```python
from build123d import *

# Parameters (mm, degrees)
SKETCH_1_R                   = 3.85
EXTRUDE_1_DEPTH              = 8
EXTRUDE_1_2_DEPTH            = 8
EXTRUDE_1_3_DEPTH            = 8
SKETCH_1_3_R                 = 28.3
SKETCH_1_3_R_2               = 0.5
EXTRUDE_2_DEPTH              = 3
SKETCH_2_R                   = 3.2
CUT_EXTRUDE_1_DEPTH          = 41.333360882
HOLE_WIZARD_M2_1_D           = 2.4
HOLE_WIZARD_M2_1_DEPTH       = 3
HOLE_WIZARD_M2_1_CBORE_D     = 5
HOLE_WIZARD_M2_1_CBORE_DEPTH = 1.6
HOLE_WIZARD_M2_1_TIP         = 0.721032743


with BuildPart() as part:
    # Sketch 1 → Extrude 1 (new body)
    with BuildSketch(Plane(origin=(0, 0, 0), x_dir=(1, 0, 0), z_dir=(0, 1, 0))):
        with Locations(Location((0, 14.33, 0), (0, 0, 270))):
            Circle(SKETCH_1_R)
    extrude(amount=EXTRUDE_1_DEPTH)



with BuildPart() as body_2:
    # Sketch 1 → Extrude 1 2 (new body)
    with BuildSketch(Plane(origin=(0, 0, 0), x_dir=(1, 0, 0), z_dir=(0, 1, 0))):
        with Locations(Location((12.410144036, -7.165, 0), (0, 0, 270))):
            Circle(SKETCH_1_R)
    extrude(amount=EXTRUDE_1_2_DEPTH)


with BuildPart() as body_3:
    # Sketch 1 → Extrude 1 3 (new body)
    with BuildSketch(Plane(origin=(0, 0, 0), x_dir=(1, 0, 0), z_dir=(0, 1, 0))):
        with Locations(Location((-12.410144036, -7.165, 0), (0, 0, 270))):
            Circle(SKETCH_1_R)
    extrude(amount=EXTRUDE_1_3_DEPTH)


with BuildPart() as part_1:
    add(part.part)

    add(body_2.part)  # Extrude 2 merges body 2

    add(body_3.part)  # Extrude 2 merges body 3
    # Sketch 1_3 → Extrude 2 (add)
    with BuildSketch(Plane(origin=(0, 0, 0), x_dir=(1, 0, 0), z_dir=(0, 1, 0))):
        with Locations(Location((0, 0, 0), (0, 0, 270))):
            Circle(SKETCH_1_3_R)
        with Locations(Location((0, -14.33, 0), (0, 0, 270))):
            Circle(SKETCH_1_3_R_2, mode=Mode.SUBTRACT)
        with Locations(Location((-12.410144036, 7.165, 0), (0, 0, 270))):
            Circle(SKETCH_1_3_R_2, mode=Mode.SUBTRACT)
        with Locations(Location((12.410144036, 7.165, 0), (0, 0, 270))):
            Circle(SKETCH_1_3_R_2, mode=Mode.SUBTRACT)
    extrude(amount=EXTRUDE_2_DEPTH)

    # Sketch 2 → Cut-Extrude 1 (cut, through all)
    with BuildSketch(Plane(origin=(0, 3, 0), x_dir=(1, 0, 0), z_dir=(0, 1, 0))):
        with Locations(Location((0, 0, 0), (0, 0, 270))):
            Circle(SKETCH_2_R)
    extrude(amount=-CUT_EXTRUDE_1_DEPTH, mode=Mode.SUBTRACT)

    # Hole Wizard M2 _ _ _ _1
    with Locations(Plane(origin=(0, 0, 0), x_dir=(-1, 0, 0), z_dir=(0, -1, 0))):
        with Locations((0, -14.33), (12.410144036, 7.165), (-12.410144036, 7.165)):
            CounterBoreHole(HOLE_WIZARD_M2_1_D / 2, HOLE_WIZARD_M2_1_CBORE_D / 2, HOLE_WIZARD_M2_1_CBORE_DEPTH, depth=HOLE_WIZARD_M2_1_DEPTH)
            with Locations((0, 0, -(HOLE_WIZARD_M2_1_DEPTH + HOLE_WIZARD_M2_1_TIP / 2))):  # 118° drill point
                Cone(0, HOLE_WIZARD_M2_1_D / 2, HOLE_WIZARD_M2_1_TIP, mode=Mode.SUBTRACT)


solid = part_1.part
```
Part model, mm, in its own coordinate system. A direction names the side the tool comes from. Round coordinates to 2 decimals unless told otherwise and drop trailing zeros. Write each loop counter-clockwise with the first axis right and the second up, starting at its lowest first coordinate (ties: lowest second). Pieces come first, ordered by that corner, then holes.
Item 1: Cut at B-B, the plane z = 0. Give the cut face in (x, y), plus the area to 3 significant figures.
Results:
outline: (-28.3, 0) - (-3.2, 0) - (-3.2, 3) - (-28.3, 3) - close; (3.2, 0) - (28.3, 0) - (28.3, 3) - (3.2, 3) - close
area: 151 mm2
Item 2: Cut at D-D, the plane z = -14.33. Give the cut face in (x, y).
Results:
outline: (-24.4, 0) - (24.4, 0) - (24.4, 3) - (3.85, 3) - (3.85, 8) - (-3.85, 8) - (-3.85, 3) - (-24.4, 3) - close
Item 3: Cut at A-A, the plane x = 0. Give the cut face in (y, z), plus the area to 3 significant figures.
Results:
outline: (0, -28.3) - (3, -28.3) - (3, -18.18) - (8, -18.18) - (8, -10.48) - (3, -10.48) - (3, -3.2) - (0, -3.2) - close; (0, 3.2) - (3, 3.2) - (3, 13.13) - (1.6, 13.13) - (1.6, 11.83) - (0, 11.83) - close; (0, 16.83) - (1.6, 16.83) - (1.6, 15.53) - (3, 15.53) - (3, 28.3) - (0, 28.3) - close
area: 178 mm2
Item 4: Cut at C-C, the plane y = 5.25. Give the cut face in (x, z) (3 decimals), plus the area to 3 significant figures.
Results:
outline: circle Ø7.7 at (-12.41, 7.165); circle Ø7.7 at (0, -14.33); circle Ø7.7 at (12.41, 7.165)
area: 140 mm2
Item 5: Which spindle directions (+Z, -Z, +X, -X, +Y, -Y) get a long thin tool onto all of the face, cutting with end or side? Do faces 1 (the cylindrical face through (16.227, 5.465, 6.664)), 2 (the cylindrical face through (11.53, 2.31, -7.98)), 3 (the cylindrical face through (0.54, 0.79, 16.77)). Say none if no direction does.
Results:
face 1: +Y
face 2: +Y, -Y
face 3: -Y
Item 6: Two-plate mould, pull along Z, no slides. Class faces 4 (the cylindrical face through (-12.085, 0.789, -9.644)), 5 (the flat face through (12, 8, 7)), 6 (the cylindrical face through (-16.17, 5.46, 6.33)): +Z half, -Z half, draft (parallel to the pull), parting line (faces both ways), or undercut.
Results:
face 4: undercut
face 5: draft
face 6: parting line
Item 7: Probe L1, parallel to X at y = 1.1, z = 0; L2, parallel to Z at x = -0.5, y = 1.75; L3, parallel to Y at x = -20.5, z = 3. List the from-to ranges inside material, lowest first.
Results:
L1: x = -28.3 to -3.2, 3.2 to 28.3
L2: z = -28.3 to -3.16, 3.16 to 13.24, 15.42 to 28.3
L3: y = 0 to 3
Item 8: Drop flat-ended pins along their axis: pin 1 Ø2.5 at (x, z) = (1, 15) entering from -Y; pin 2 Ø1.4 at (x, z) = (-12.41, -7.16) entering from -Y; pin 3 Ø4 at (x, z) = (18.5, -20) entering from +Y; pin 4 Ø1.5 at (x, y) = (12.5, 1) entering from -Z. Give the stop position or say it passes through.
Results:
pin 1: stops at y = 1.6
pin 2: passes through
pin 3: stops at y = 3
pin 4: stops at z = -25.75
